Here's how the part is built. I have some questions about the finished solid (model axes, mm). Round coordinates to 2 decimals unless told otherwise and drop trailing zeros. Loops run counter-clockwise (first coordinate to the right, second up) from the corner with the lowest first, then second, coordinate; pieces in that order, holes last. Notation, with made-up numbers: M 34,71 L 75,71 A16 ccw 75,88 Z; hole C 3.25,19 d11. An arc over 180 degrees is marked long. Use a Markdown table: item, result.
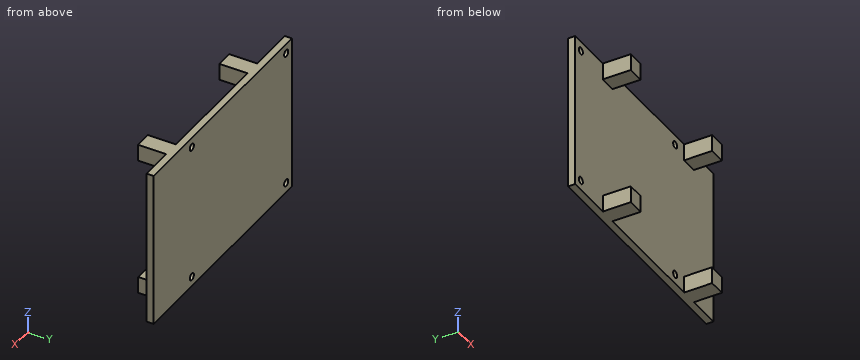
from build123d import *

# Parameters (mm, degrees)
SKETCH1_W                   = 85
SKETCH1_H                   = 56
BOSS_EXTRUDE1_DEPTH         = 2.5
TAP_DRILL_FOR_M3X0_5_TAP2_D = 2.5
SKETCH5_W                   = 6
SKETCH5_H                   = 6
BOSS_EXTRUDE2_DEPTH         = 10


with BuildPart() as part:
    # Sketch1 → Boss-Extrude1 (new body)
    with BuildSketch(Plane(origin=(0, 0, 0), x_dir=(1, 0, 0), z_dir=(0, 1, 0))):
        with Locations((42.5, -28)):
            Rectangle(SKETCH1_W, SKETCH1_H)
    extrude(amount=BOSS_EXTRUDE1_DEPTH)

    # Tap Drill for M3x0.5 Tap2 (through all)
    with Locations(Plane(origin=(0, 2.5, 0), x_dir=(1, 0, 0), z_dir=(0, 1, 0))):
        with Locations((3.5, -3.5), (61.5, -3.5), (61.5, -52.5), (3.5, -52.5)):
            Hole(TAP_DRILL_FOR_M3X0_5_TAP2_D / 2)

    # Sketch5 → Boss-Extrude2 (add)
    with BuildSketch(Plane.XZ):
        with Locations((20, 3)):
            Rectangle(SKETCH5_W, SKETCH5_H)
        with Locations((20, 53)):
            Rectangle(SKETCH5_W, SKETCH5_H)
        with Locations((70, 3)):
            Rectangle(SKETCH5_W, SKETCH5_H)
        with Locations((70, 53)):
            Rectangle(SKETCH5_W, SKETCH5_H)
    extrude(amount=BOSS_EXTRUDE2_DEPTH)


solid = part.part
1. I need wall thicknesses on probe 1 along X at (y, z) = (0.95, 52.5); probe 2 along Z at (x, y) = (3.5, 2); probe 3 along Y at (x, z) = (69.5, 28.5). Which ranges of each line are inside material? Lowest first, please. Write a range as from..to.
Answer sheet:
| item | result |
|---|---|
| probe 1 | 0..2.25, 4.75..60.25, 62.75..85 |
| probe 2 | 0..2.25, 4.75..51.25, 53.75..56 |
| probe 3 | 0..2.5 |
2. Imagine slicing it at A-A, the plane y = -2. Write out the boundary of the cut face in (x, z), then the cut area to 3 significant figures.
Answer sheet:
| item | result |
|---|---|
| outline | M 17,0 L 23,0 L 23,6 L 17,6 Z; M 17,50 L 23,50 L 23,56 L 17,56 Z; M 67,0 L 73,0 L 73,6 L 67,6 Z; M 67,50 L 73,50 L 73,56 L 67,56 Z |
| area | 144 mm2 |
3. Imagine slicing it at B-B, the plane z = 3.5. Write out the boundary of the cut face in (x, y).
Answer sheet:
| item | result |
|---|---|
| outline | M 0,0 L 2.25,0 L 2.25,2.5 L 0,2.5 Z; M 4.75,0 L 17,0 L 17,-10 L 23,-10 L 23,0 L 60.25,0 L 60.25,2.5 L 4.75,2.5 Z; M 62.75,0 L 67,0 L 67,-10 L 73,-10 L 73,0 L 85,0 L 85,2.5 L 62.75,2.5 Z |
4. Imagine slicing it at D-D, the plane z = 35.5. Write out the boundary of the cut face in (x, y).
Answer sheet:
| item | result |
|---|---|
| outline | M 0,0 L 85,0 L 85,2.5 L 0,2.5 Z |
5. Imagine slicing it at C-C, the plane x = 61.5. Write out the boundary of the cut face in (y, z), then the cut area to 4 significant figures.
Answer sheet:
| item | result |
|---|---|
| outline | M 0,0 L 2.5,0 L 2.5,2.25 L 0,2.25 Z; M 0,4.75 L 2.5,4.75 L 2.5,51.25 L 0,51.25 Z; M 0,53.75 L 2.5,53.75 L 2.5,56 L 0,56 Z |
| area | 127.5 mm2 |
6. For pin 1 Ø6 at (y, z) = (-1, 10) entering from +X; pin 2 Ø6.5 at (y, z) = (-3.5, 1.5) entering from +X; pin 3 Ø1.8 at (y, z) = (-4.5, 52.5) entering from -X; pin 4 Ø10 at (x, z) = (73, 27) entering from -Y, each with a flat end and sliding along its axis, tell me the tip position at first contact or that it passes through.
Answer sheet:
| item | result |
|---|---|
| pin 1 | x = 85 |
| pin 2 | x = 73 |
| pin 3 | x = 17 |
| pin 4 | y = 0 |
